```python
from build123d import *

# Parameters (mm, degrees)
SKETCH_1_R          = 16
EXTRUDE_1_DEPTH     = 6
SKETCH_4_R          = 3
CUT_EXTRUDE_2_DEPTH = 24.409399821


with BuildPart() as part:
    # Эскиз1 → Вытянуть1 (new body)
    with BuildSketch(Plane(origin=(0, 0, 0), x_dir=(1, 0, 0), z_dir=(0, 1, 0))):
        with Locations(Location((0, 0, 0), (0, 0, 270))):
            Circle(SKETCH_1_R)
    extrude(amount=EXTRUDE_1_DEPTH)

    # Эскиз2 → Вырез-Повернуть1 (revolve, cut)
    with BuildSketch(Plane.XY, mode=Mode.PRIVATE) as cut_revolve_1_sk:
        with BuildLine():
            Line((16, 0.7), (13.508420421, 2.60261237))
            ThreePointArc((13.508420421, 2.60261237), (13.311872347, 3), (13.508420421, 3.39738763))
            Line((13.508420421, 3.39738763), (16, 5.3))
            Line((16, 5.3), (16, 0.7))
        make_face()
    revolve(cut_revolve_1_sk.sketch.rotate(Axis((0, 0, 0), (0, 1, 0)), 90), axis=Axis((0, 0, 0), (0, 1, 0)), mode=Mode.SUBTRACT)

    # Эскиз4 → Вытянуть2 (cut, through all)
    with BuildSketch(Plane(origin=(0, 6, 0), x_dir=(1, 0, 0), z_dir=(0, 1, 0))):
        with Locations(Location((0, 0, 0), (0, 0, 270))):
            Circle(SKETCH_4_R)
    extrude(amount=-CUT_EXTRUDE_2_DEPTH, mode=Mode.SUBTRACT)


solid = part.part
```
Design review of the part built by this model. Coordinates are the model's own, in mm. A direction names the side the tool comes from. Round coordinates to 2 decimals unless told otherwise and drop trailing zeros. Write each loop counter-clockwise with the first axis right and the second up, starting at its lowest first coordinate (ties: lowest second). Pieces come first, ordered by that corner, then holes. Notation, with made-up numbers: (19.5, -21) -> (40.5, -21) arc R21 ccw to (40.5, -7) -> close; hole circle Ø2 at (-26, 14). An arc over 180 degrees is marked (long way). Write item = value, one per line. Start each with the question number.
1) Mouldability with a two-part tool opening along Y and no side actions: class faces 3 (the face through (-3.3, 0, -0.2)), 4 (the face through (-3.3, 6, -0.2)), 5 (the face through (13.339, 3.516, 2.962)) as +Y half, -Y half, draft (parallel to the pull), parting line (faces both ways), or undercut.
2) Wall thickness on probe 1 along X at (y, z) = (2.2, 0); probe 2 along X at (y, z) = (5.35, 0); probe 3 along Y at (x, z) = (11, -9.5): over which ranges is each line inside the solid? List them lowest first. Write a range as from..to.
3) Take a section at A-A, the plane x = 0. State the section outline as (y, z) points, plus the area to 3 significant figures.
4) Clearance check with flat-ended pins moving along their axes: pin 1 (2 mm diameter, centred on x = 10.5, y = 5, fed in from +Z); pin 2 (2 mm diameter, centred on x = -9.5, y = 3.5, fed in from +Z); pin 3 (1.5 mm diameter, centred on y = 5, z = -4.5, fed in from +X). State where each tip first meets the part, or that it passes through.
5) Take a section at B-B, the plane z = 0. State the section outline as (x, y) points.
6) Tool access review of faces 1 (the face through (-4.09, 2.51, -13)), 2 (the face through (-15.62, 5.65, -3.47)): name each direction out of +Z, -Z, +X, -X, +Y, -Y from which nothing blocks a thin tool from reaching the whole face with its end or side.
Results list:
q1.face_3 = -Y half
q1.face_4 = +Y half
q1.face_5 = undercut
q2.probe_1 = -14.04..-3, 3..14.04
q2.probe_2 = -16..-3, 3..16
q2.probe_3 = 0..1.82, 4.18..6
q3.outline = (0, -16) -> (0.7, -16) -> (2.6, -13.51) arc R0.5 cw to (3.4, -13.51) -> (5.3, -16) -> (6, -16) -> (6, -3) -> (0, -3) -> close; (0, 3) -> (6, 3) -> (6, 16) -> (5.3, 16) -> (3.4, 13.51) arc R0.5 cw to (2.6, 13.51) -> (0.7, 16) -> (0, 16) -> close
q3.area = 142 mm²
q4.pin_1 = 12.84
q4.pin_2 = 11.73
q4.pin_3 = 15.54
q5.outline = (-16, 0) -> (-3, 0) -> (-3, 6) -> (-16, 6) -> (-16, 5.3) -> (-13.51, 3.4) arc R0.5 cw to (-13.51, 2.6) -> (-16, 0.7) -> close; (3, 0) -> (16, 0) -> (16, 0.7) -> (13.51, 2.6) arc R0.5 cw to (13.51, 3.4) -> (16, 5.3) -> (16, 6) -> (3, 6) -> close
q6.face_1 = none
q6.face_2 = +Y, -Y
